from build123d import *

# Parameters (mm, degrees)
BOSS_EXTRUDE1_DEPTH  = 100
BOSS_EXTRUDE2_REACH  = 207.357
SKETCH6_R            = 12.5
SKETCH6_R_2          = 6
BOSS_EXTRUDE4_DEPTH  = 15
SKETCH7_R            = 6
CUT_EXTRUDE3_DEPTH   = 206.356636358
BOSS_EXTRUDE10_REACH = 190.828
CUT_EXTRUDE6_DEPTH   = 5


with BuildPart() as part:
    # Sketch1 → Boss-Extrude1 (new body)
    with BuildSketch(Plane.XY):
        Polygon((-177.777777778, 0), (-177.777777778, 25), (-77.777777778, 25), (-37.777777778, 40), (22.222222222, 40), (22.222222222, 0), (-27.777777778, 0), (-27.777777778, -10), (-65.277777778, -10), (-65.277777778, 0), (-90.277777778, 0), (-90.277777778, -10), (-127.777777778, -10), (-127.777777778, 0), align=None)
    extrude(amount=BOSS_EXTRUDE1_DEPTH)

    # Sketch5 → Boss-Extrude2 (add, up to next)
    with BuildSketch(Plane(origin=(0, 54.214936023, 19.732622965), x_dir=(-1, 0, 0), z_dir=(0, 0.939692620785908, 0.34202014332566977)), mode=Mode.PRIVATE) as boss_extrude2_sk1:
        with BuildLine():
            Line((112.777777778, 85.418758495), (112.777777778, 45.418758495))
            ThreePointArc((112.777777778, 45.418758495), (137.777777778, 20.418758495), (162.777777778, 45.418758495))
            Line((162.777777778, 45.418758495), (162.777777778, 85.418758495))
            Line((162.777777778, 85.418758495), (112.777777778, 85.418758495))
        make_face()
    boss_extrude2_tool1 = extrude(boss_extrude2_sk1.sketch, amount=-BOSS_EXTRUDE2_REACH, mode=Mode.PRIVATE) - part.part
    add(boss_extrude2_tool1.solids().sort_by_distance((-137.777778, 35.287462, 71.735431))[0])

    # Sketch6 → Boss-Extrude4 (add)
    with BuildSketch(Plane(origin=(0, 54.214936023, 19.732622965), x_dir=(1, 0, 0), z_dir=(0, 0.9396926207859081, 0.3420201433256699))):
        with Locations(Location((-137.777777778, -45.418758495, 0), (0, 0, 270))):
            Circle(SKETCH6_R)
        with Locations(Location((-137.777777778, -45.418758495, 0), (0, 0, 270))):
            Circle(SKETCH6_R_2, mode=Mode.SUBTRACT)
    extrude(amount=BOSS_EXTRUDE4_DEPTH)

    # Sketch7 → Cut-Extrude3 (cut, through all)
    with BuildSketch(Plane(origin=(0, 54.214936023, 19.732622965), x_dir=(1, 0, 0), z_dir=(0, 0.9396926207859081, 0.3420201433256699))):
        with Locations(Location((-137.777777778, -45.418758495, 0), (0, 0, 270))):
            Circle(SKETCH7_R)
    extrude(amount=-CUT_EXTRUDE3_DEPTH, mode=Mode.SUBTRACT)

    # Sketch10 → Boss-Extrude10 (add, up to next)
    with BuildSketch(Plane(origin=(-30.269761992, 52.428765703, 0), x_dir=(0, 0, -1), z_dir=(-0.5000000000000012, 0.8660254037844379, 0)), mode=Mode.PRIVATE) as boss_extrude10_sk1:
        with BuildLine():
            Line((-69.661280828, 54.857531405), (-69.661280828, 4.857531405))
            ThreePointArc((-69.661280828, 4.857531405), (-37.095944154, -30.057686115), (0, 0))
            Line((0, 0), (0, 54.857531405))
            Line((0, 54.857531405), (-69.661280828, 54.857531405))
        make_face()
    boss_extrude10_tool1 = extrude(boss_extrude10_sk1.sketch, amount=-BOSS_EXTRUDE10_REACH, mode=Mode.PRIVATE) - part.part
    add(boss_extrude10_tool1.solids().sort_by_distance((-43.846947, 44.589974, 34.777462))[0])

    # Sketch11 → Cut-Extrude6 (cut)
    with BuildSketch(Plane(origin=(-30.269761992, 52.428765703, 0), x_dir=(0.866025403784438, 0.5000000000000012, 0), z_dir=(-0.5000000000000011, 0.8660254037844379, 0))):
        with BuildLine():
            Line((-54.857531405, -34.830640414), (-54.831038967, -39.830570229))
            Line((-54.831038967, -39.830570229), (-16.329059293, -39.626565102))
            ThreePointArc((-16.329059293, -39.626565102), (-13.709739092, -43.486722407), (-9.857531405, -46.117720065))
            Line((-9.857531405, -46.117720065), (-9.857531405, -69.661280828))
            Line((-9.857531405, -69.661280828), (-4.857531405, -69.661280828))
            ThreePointArc((-4.857531405, -69.661280828), (-2.351096218, -69.571419508), (0.142468595, -69.302296979))
            Line((0.142468595, -69.302296979), (0.142468595, -46.117720065))
            ThreePointArc((0.142468595, -46.117720065), (4.041313515, -43.439695211), (6.665968636, -39.50472452))
            Line((6.665968636, -39.50472452), (29.822643788, -39.382027441))
            ThreePointArc((29.822643788, -39.382027441), (30.065429756, -36.982225405), (30.142353187, -34.571400312))
            Line((30.142353187, -34.571400312), (30.141340464, -34.380268592))
            ThreePointArc((30.141340464, -34.380268592), (30.031317876, -31.874132501), (29.742071325, -29.382313987))
            Line((29.742071325, -29.382313987), (6.529563607, -29.505306898))
            ThreePointArc((6.529563607, -29.505306898), (3.92074784, -25.762302601), (0.142468595, -23.204841591))
            Line((0.142468595, -23.204841591), (0.142468595, -0.020264677))
            ThreePointArc((0.142468595, -0.020264677), (0.071244712, -0.010059118), (0, 0))
            Line((0, 0), (-9.857531405, 0))
            Line((-9.857531405, 0), (-9.857531405, -23.204841591))
            ThreePointArc((-9.857531405, -23.204841591), (-13.682838556, -25.808939121), (-16.298624018, -29.626263466))
            Line((-16.298624018, -29.626263466), (-54.857531405, -29.830570228))
            Line((-54.857531405, -29.830570228), (-54.857531405, -34.830640414))
        make_face()
    extrude(amount=-CUT_EXTRUDE6_DEPTH, mode=Mode.SUBTRACT)


solid = part.part
Read the model definition and answer for the solid it produces. Units are mm, in the model's axes. A direction names the side the tool comes from. Round coordinates to 2 decimals unless told otherwise and drop trailing zeros. Order: outer loops, then holes, each group sorted by start corner. A loop starts at its lowest first (then second) coordinate and runs counter-clockwise, first axis right, second up.
1) The part is cut by section B-B on z = 13.5. Write down the section's boundary in (x, y).
2) The part is cut by section C-C on y = 27. Give the number of separate pieces and of enclosed holes in the cut face, plus the area to 3 significant figures.
3) The mould has two halves that part along Y. Classify faces 1 (the face through (-58.57, 36.09, 15.12)), 2 (the face through (-177.778, 12, 49)), 3 (the face through (-25.6, 52.28, 25.81)): released by +Y, released by -Y, zero draft, split by the parting line, or undercut.
4) Straight lines are drawn through the part: L1, parallel to X at y = -5, z = 25.5; L2, parallel to Y at x = -4, z = 94.5; L3, parallel to X at y = 26, z = 68. For each, find the intervals that lie inside material, in ascending order.
5) The part is cut by section A-A on y = -2. Write down the section's boundary in (x, z), plus the area to 3 significant figures.
6) The part is cut by section D-D on x = -148. Write down the section's boundary in (y, z).
7) For faces 4 (the face through (-127.778, -5, 49)), 5 (the face through (-48, 38, 69.661)), 6 (the face through (-58.57, 36.09, 56.36)), 7 (the face through (-78, 0, 49)), determine the directions among +Z, -Z, +X, -X, +Y, -Y from which every point of the face is accessible in a straight line to the end or side of a thin tool.
8) Flat-ended cylindrical pins translate along their axes: pin 1 (8 mm diameter, centred on y = -6, z = 67.5, fed in from -X); pin 2 (7.5 mm diameter, centred on x = -81.5, z = 41, fed in from -Y); pin 3 (10 mm diameter, centred on x = -101.5, z = 43.5, fed in from +Y). Find the tip coordinate at first contact, or state that the pin passes through.
Resolved:
1. outline: (-177.78, 0) - (-127.78, 0) - (-127.78, -10) - (-90.28, -10) - (-90.28, 0) - (-65.28, 0) - (-65.28, -10) - (-27.78, -10) - (-27.78, 0) - (22.22, 0) - (22.22, 40) - (3.49, 40) - (-10.33, 63.94) - (-30.15, 52.5) - (-27.65, 48.17) - (-36.31, 43.17) - (-38.81, 47.5) - (-77.78, 25) - (-177.78, 25) - close
2. separate pieces: 2
2. enclosed holes: 1
2. area: 12,200 mm2
3. face 1: released by +Y
3. face 2: zero draft
3. face 3: undercut
4. L1: x = -127.78 to -90.28, -65.28 to -27.78
4. L2: y = 0 to 40
4. L3: x = -162.78 to -112.78, -76.05 to 22.22
5. outline: (-127.78, 0) - (-90.28, 0) - (-90.28, 100) - (-127.78, 100) - close; (-65.28, 0) - (-27.78, 0) - (-27.78, 100) - (-65.28, 100) - close
5. area: 7,500 mm2
6. outline: (0, 0) - (25, 0) - (25, 33.15) - (46.48, 40.97) - (41.14, 55.65) - (55.24, 60.78) - (50.32, 74.3) - (36.22, 69.17) - (25, 100) - (0, 100) - close
7. face 4: +Z, -Z, -X, -Y
7. face 5: +Z, +Y
7. face 6: +Z, -Z, +Y
7. face 7: +Z, -Z, -Y
8. pin 1: stops at x = -127.78
8. pin 2: stops at y = 0
8. pin 3: stops at y = 25
